Part model, mm, in its own coordinate system. Face numbers are marked on the shaded views. Round coordinates to 2 decimals unless told otherwise and drop trailing zeros. Order: outer loops, then holes, each group sorted by start corner. A loop starts at its lowest first (then second) coordinate and runs counter-clockwise, first axis right, second up. Notation, with made-up numbers: (-28, 31) -> (-3, 31) arc R24 ccw to (-3, 50) -> close; hole circle Ø5 at (-11.5, 3.5). An arc over 180 degrees is marked (long way). Return JSON: item names as keys, results as strings. Group by question number.
from build123d import *

# Parameters (mm, degrees)
F0_R     = 13
F1_DEPTH = 4


with BuildPart() as f1:
    # F0 (on Right) → F1 (new body)
    with BuildSketch(Plane.YZ):
        Polygon((15.412828, -15.937231), (-22.950384, -15.937231), (-22.950384, -17.937231), (15.699004, -17.937231), align=None)
        Polygon((-22.950384, 20.790322), (-22.950384, -15.937231), (15.412828, -15.937231), (15.679364, 16.999187), (17.621164, 20.790322), (10.5, 20.790322), (8.581838, 20.790322), (10.5, 18.970987), (10.5, 13.970987), (-10.5, 13.970987), (-10.5, 18.970987), (-10.25, 20.790322), (-18.572044, 20.790322), (-18.572044, 3.790322), (-20.572044, 3.790322), (-20.572044, 20.790322), align=None)
        Circle(F0_R, mode=Mode.SUBTRACT)
    extrude(amount=F1_DEPTH)


solid = f1.part
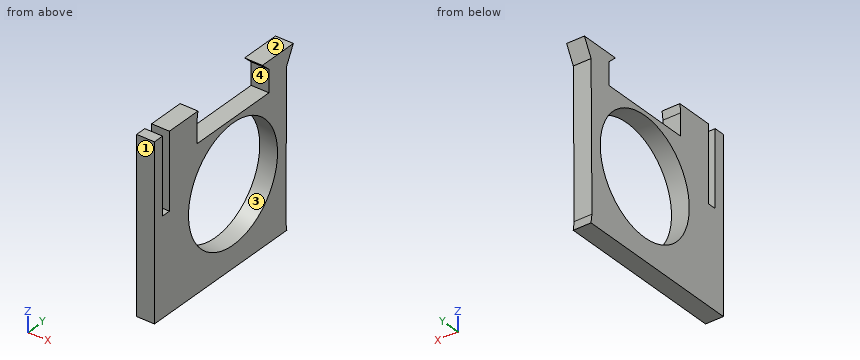
(1) Saw through at A-A, the plane x = 3.25. List the corners of the cut face in (y, z), and give its area (3 significant figures).
(2) Saw through at B-B, the plane y = 0. List the corners of the cut face in (x, z), and give its area (3 significant figures).
(3) Probe L1, parallel to Z at x = 1.35, y = 0; L2, parallel to Z at x = 3.5, y = -5; L3, parallel to Y at x = 3.1, z = -14.5. List the from-to ranges inside material, lowest first. Write a range as [from, to].
(4) Pin check, flat tips, straight feed: P1, Ø2, axis at x = 1.5, z = 15.5, coming from the +Y side; P2, Ø0.6, axis at x = 2, y = -19, coming from the +Z side; P3, Ø2, axis at x = 1.5, z = 9.5, coming from the +Y side; P4, Ø6, axis at y = 2.5, z = -9.5, coming from the -X side. Stop position of each tip, or through.
(5) Saw through at C-C, the plane z = -7. List the corners of the cut face in (x, y), and give its area (3 significant figures).
(6) Mould opens along Y. For the marked faces 1, 2, 3 and 4 say: pulls with the +Y half, pulls with the -Y half, needs draft (parallel to the pull), parting line crosses it, or undercut.
Results are:
{
 "1": {"outline": "(-22.95, -17.94) -> (15.7, -17.94) -> (15.41, -15.94) -> (15.68, 17) -> (17.62, 20.79) -> (8.58, 20.79) -> (10.5, 18.97) -> (10.5, 13.97) -> (-10.5, 13.97) -> (-10.5, 18.97) -> (-10.25, 20.79) -> (-18.57, 20.79) -> (-18.57, 3.79) -> (-20.57, 3.79) -> (-20.57, 20.79) -> (-22.95, 20.79) -> close; hole circle Ø26 at (0, 0)", "area": "789 mm^2"},
 "2": {"outline": "(0, -17.94) -> (4, -17.94) -> (4, -13) -> (0, -13) -> close; (0, 13) -> (4, 13) -> (4, 13.97) -> (0, 13.97) -> close", "area": "23.6 mm^2"},
 "3": {"L1": "z = [-17.94, -13], [13, 13.97]", "L2": "z = [-17.94, -12], [12, 13.97]", "L3": "y = [-22.95, 15.42]"},
 "4": {"P1": "stops at y = 15.68", "P2": "stops at z = 3.79", "P3": "stops at y = 15.63", "P4": "passes through"},
 "5": {"outline": "(0, -22.95) -> (4, -22.95) -> (4, -10.95) -> (0, -10.95) -> close; (0, 10.95) -> (4, 10.95) -> (4, 15.49) -> (0, 15.49) -> close", "area": "66.1 mm^2"},
 "6": {"face 1": "pulls with the -Y half", "face 2": "needs draft", "face 3": "undercut", "face 4": "undercut"}
}
